Geometry: see drawing. Coordinates: mm, zero at the bounding-box minimum. A direction names the side the tool comes from. Round coordinates to 2 decimals unless told otherwise and drop trailing zeros. Order: outer loops, then holes, each group sorted by start corner. A loop starts at its lowest first (then second) coordinate and runs counter-clockwise, first axis right, second up. Notation, with made-up numbers: (-35.5, 18.25) -> (1.5, 18.25) arc R12 ccw to (1.5, 38.25) -> close; hole circle Ø7 at (4.25, -17.5). An arc over 180 degrees is marked (long way). Use a Markdown table: item, result.
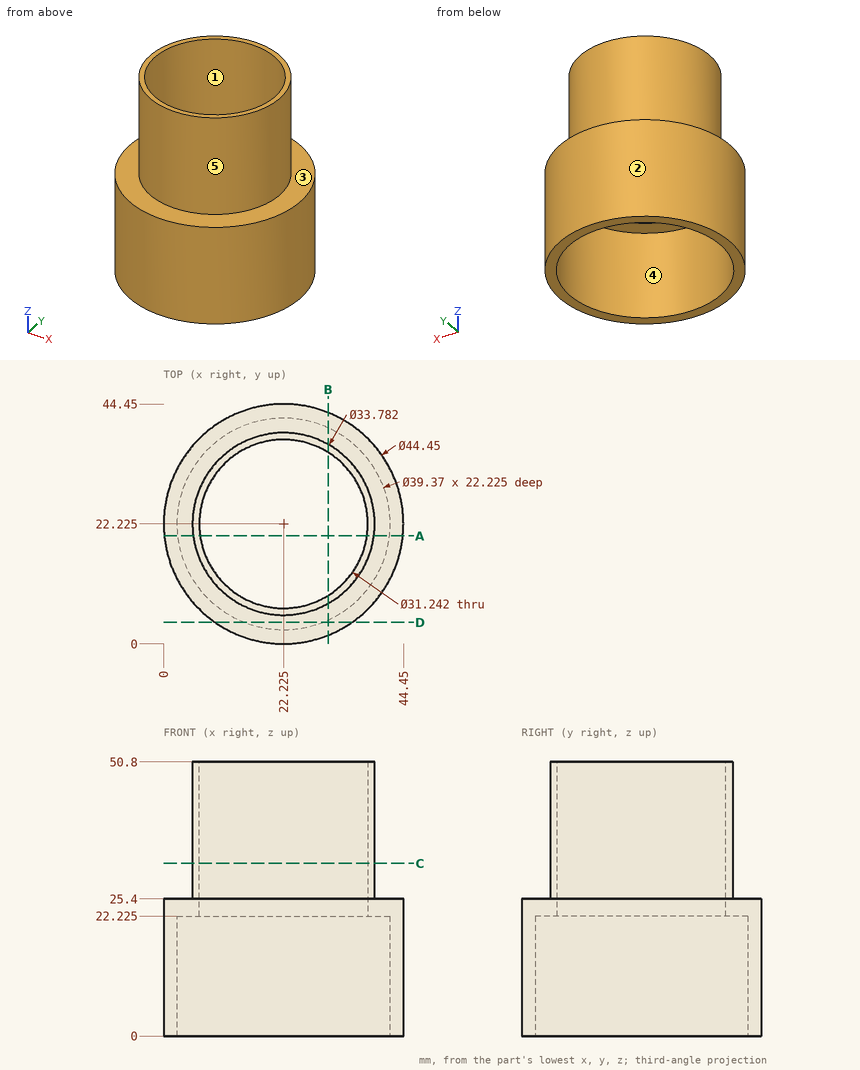
1) Contact query for flat-ended pins moving along their axis: P1, Ø6, axis at x = 34, z = 20.5, coming from the +Y side; P2, Ø10, axis at y = 10, z = 12, coming from the +X side; P3, Ø2, axis at x = 38, z = 16, coming from the -Y side. Output: stop coordinate, or through.
Answer key:
| item | result |
|---|---|
| P1 | stops at y = 42.64 |
| P2 | stops at x = 43.24 |
| P3 | stops at y = 5.62 |
2) Cut plane A-A on y = 20. Return loops of the section in (x, z) (3 decimals), and give its area (3 significant figures).
Answer key:
| item | result |
|---|---|
| outline | (0.112, 0) -> (2.666, 0) -> (2.666, 22.225) -> (6.763, 22.225) -> (6.763, 50.8) -> (5.481, 50.8) -> (5.481, 25.4) -> (0.112, 25.4) -> close; (37.687, 22.225) -> (41.784, 22.225) -> (41.784, 0) -> (44.338, 0) -> (44.338, 25.4) -> (38.969, 25.4) -> (38.969, 50.8) -> (37.687, 50.8) -> close |
| area | 221 mm^2 |
3) Set-up query: the marked faces 4 and 5. Return all of +Z, -Z, +X, -X, +Y, -Y with unobstructed straight access to the full face (end or side cutting, diameter ignored); none if empty.
Answer key:
| item | result |
|---|---|
| face 4 | -Z |
| face 5 | +Z |
4) Ray query, probe 1 along X at (y, z) = (22, 44); probe 2 along Y at (x, z) = (21.5, 15); probe 3 along X at (y, z) = (12.5, 5). Return the intervals inside material, ascending.
Answer key:
| item | result |
|---|---|
| probe 1 | x = 5.34 to 6.61, 37.84 to 39.11 |
| probe 2 | y = 0.01 to 2.55, 41.9 to 44.44 |
| probe 3 | x = 2.24 to 5.11, 39.34 to 42.21 |
5) Cut plane D-D on y = 4. Return loops of the section in (x, z) (3 decimals).
Answer key:
| item | result |
|---|---|
| outline | (9.505, 0) -> (14.785, 0) -> (14.785, 22.225) -> (29.665, 22.225) -> (29.665, 0) -> (34.945, 0) -> (34.945, 25.4) -> (9.505, 25.4) -> close |
6) Draft query along X for the marked faces 1, 2 and 3. Return one class per face: released by +X, released by -X, zero draft, split by the parting line, or undercut.
Answer key:
| item | result |
|---|---|
| face 1 | undercut |
| face 2 | split by the parting line |
| face 3 | zero draft |
7) Cut plane C-C on z = 32. Return loops of the section in (x, y) (3 decimals).
Answer key:
| item | result |
|---|---|
| outline | circle Ø33.782 at (22.225, 22.225); hole circle Ø31.242 at (22.225, 22.225) |
8) Cut plane B-B on x = 30.5. Return loops of the section in (y, z) (3 decimals).
Answer key:
| item | result |
|---|---|
| outline | (1.598, 0) -> (4.364, 0) -> (4.364, 22.225) -> (8.976, 22.225) -> (8.976, 50.8) -> (7.5, 50.8) -> (7.5, 25.4) -> (1.598, 25.4) -> close; (35.474, 22.225) -> (40.086, 22.225) -> (40.086, 0) -> (42.852, 0) -> (42.852, 25.4) -> (36.95, 25.4) -> (36.95, 50.8) -> (35.474, 50.8) -> close |
